```python
from build123d import *

# Parameters (mm, degrees)
F0_W     = 1235.329
F0_H     = 1610.36
F0_W_2   = 203.2
F0_H_2   = 76.2
F1_DEPTH = 758.444
F2_W     = 628.904
F2_H     = 203.2
F3_DEPTH = 1235.33
F5_DEPTH = 71.12
F6_R     = 9.525
F6_R_2   = 17.4625
F6_R_3   = 20.6375
F7_DEPTH = 63.5


with BuildPart() as f1:
    # F0 (on Front) → F1 (new body)
    with BuildSketch(Plane.XZ):
        with Locations((617.6645, 805.18)):
            Rectangle(F0_W, F0_H)
        with Locations((294.64, 50.8)):
            Rectangle(F0_W_2, F0_H_2, mode=Mode.SUBTRACT)
        with Locations((940.689, 50.8)):
            Rectangle(F0_W_2, F0_H_2, mode=Mode.SUBTRACT)
    extrude(amount=F1_DEPTH)

    # F2 (on face) → F3 (cut, through all)
    with BuildSketch(Plane(origin=(0, 0, 0), x_dir=(0, -1, 0), z_dir=(-1, 0, 0))):
        with Locations((379.222, -5.842)):
            Rectangle(F2_W, F2_H)
    extrude(amount=-F3_DEPTH, mode=Mode.SUBTRACT)

    # F4 (on face) → F5 (join)
    with BuildSketch(Plane.XY.offset(1610.36)):
        Polygon((435.080191, -632.46), (612.14, -455.400191), (612.14, -204.999809), (435.080191, -27.94), (184.679809, -27.94), (7.62, -204.999809), (7.62, -455.400191), (184.679809, -632.46), align=None)
        Polygon((1050.649191, -632.46), (1227.709, -455.400191), (1227.709, -204.999809), (1050.649191, -27.94), (800.248809, -27.94), (623.189, -204.999809), (623.189, -455.400191), (800.248809, -632.46), align=None)
    extrude(amount=F5_DEPTH)

    # F6 (on face) → F7 (join)
    with BuildSketch(Plane.XZ.offset(758.444)):
        with Locations((1062.99, 224.79)):
            Circle(F6_R)
        with Locations((1113.79, 193.04)):
            Circle(F6_R_2)
        with Locations((1062.99, 167.64)):
            Circle(F6_R_3)
    extrude(amount=F7_DEPTH)


solid = f1.part
```
Check sheet for the modelled part. Datum: model origin and axes. Units: mm. A direction names the side the tool comes from. Round coordinates to 2 decimals unless told otherwise and drop trailing zeros. Order: outer loops, then holes, each group sorted by start corner. A loop starts at its lowest first (then second) coordinate and runs counter-clockwise, first axis right, second up. Notation, with made-up numbers: (-18.75, 19.5) -> (20.25, 19.5) arc R25 cw to (20.25, 34.5) -> close; hole circle Ø10 at (7.5, 6.5). An arc over 180 degrees is marked (long way). One line per item, written item: value. Start each with the question number.
Q1. Thickness scan on line 1 (Z direction, x = 877, y = -751.5); line 2 (Y direction, x = 1019, z = 1599.5); line 3 (Z direction, x = 391, y = -141). Record the ranges inside material, lowest first.
Q2. Cross-section at C-C (x = 712.5). Record the boundary of the cut face in (y, z).
Q3. Cross-section at D-D (z = 1217). Record the boundary of the cut face in (x, y).
Q4. Cross-section at A-A (x = 940.5). Record the boundary of the cut face in (y, z), and give its area (3 significant figures).
Q5. Cross-section at B-B (y = -333). Record the boundary of the cut face in (x, z), and give its area (3 significant figures).
Q6. Gauge pin test, flat end, axial feed: pin 1 Ø10 at (x, y) = (864.5, -200.5) entering from -Z. Record the tip position at first contact, or that the pin passes through.
Q7. Set-up check for faces 1 (the face through (710.48, -542.69, 1645.42)), 2 (the face through (612.14, -332, 1645)), 3 (the face through (293, -726, 88.9)), 4 (the face through (609, -375, 95.758)): record each of +Z, -Z, +X, -X, +Y, -Y from which the full face is reachable in a straight line by a thin tool's end or side.
Q8. Mould release check, pull along Z, two halves, no side actions. Record for faces 5 (the face through (7.62, -328, 1645)), 6 (the face through (939, -32, 12.7)), 7 (the face through (609, -32, 0)): pulls with the +Z half, pulls with the -Z half, needs draft (parallel to the pull), parting line crosses it, or undercut.
Completed:
1. line 1: z = 0 to 12.7, 88.9 to 1610.36
1. line 2: y = -758.44 to 0
1. line 3: z = 95.76 to 1681.48
2. outline: (-758.44, 0) -> (-693.67, 0) -> (-693.67, 95.76) -> (-64.77, 95.76) -> (-64.77, 0) -> (0, 0) -> (0, 1610.36) -> (-115.69, 1610.36) -> (-115.69, 1681.48) -> (-544.71, 1681.48) -> (-544.71, 1610.36) -> (-758.44, 1610.36) -> close
3. outline: (0, -758.44) -> (1235.33, -758.44) -> (1235.33, 0) -> (0, 0) -> close
4. outline: (-758.44, 0) -> (-693.67, 0) -> (-693.67, 12.7) -> (-758.44, 12.7) -> close; (-758.44, 88.9) -> (-693.67, 88.9) -> (-693.67, 95.76) -> (-64.77, 95.76) -> (-64.77, 88.9) -> (0, 88.9) -> (0, 1610.36) -> (-27.94, 1610.36) -> (-27.94, 1681.48) -> (-632.46, 1681.48) -> (-632.46, 1610.36) -> (-758.44, 1610.36) -> close; (-64.77, 0) -> (0, 0) -> (0, 12.7) -> (-64.77, 12.7) -> close
4. area: 1,190,000 mm²
5. outline: (0, 95.76) -> (1235.33, 95.76) -> (1235.33, 1610.36) -> (1227.71, 1610.36) -> (1227.71, 1681.48) -> (623.19, 1681.48) -> (623.19, 1610.36) -> (612.14, 1610.36) -> (612.14, 1681.48) -> (7.62, 1681.48) -> (7.62, 1610.36) -> (0, 1610.36) -> close
5. area: 1,960,000 mm²
6. pin 1: stops at z = 95.76
7. face 1: +Z, -Y
7. face 2: +Z, +Y, -Y
7. face 3: +Y, -Y
7. face 4: -Z, +X, -X
8. face 5: needs draft
8. face 6: undercut
8. face 7: pulls with the -Z half
